from build123d import *

# Parameters (mm, degrees)
F1_DEPTH = 30
F3_R     = 3


# Not quite as in the source:
# - a feature of the source that left no trace in its solid (it failed there, or was rolled back) is left out


with BuildPart() as f1:
    # F0 (on Top) → F1 (new body)
    with BuildSketch(Plane.XY):
        with BuildLine():
            ThreePointArc((-37.25, 36.5), (-27.8459144936, 7.7690354349), (0, -4))
            ThreePointArc((0, -4), (26.5127811208, 8.5143386541), (35.25, 36.5))
            Line((35.25, 36.5), (-37.25, 36.5))
        make_face()
        with BuildLine():
            ThreePointArc((0, 0), (-23.5433609961, 9.1719845194), (-33.25, 32.5))
            Line((-33.25, 32.5), (31.25, 32.5))
            ThreePointArc((31.25, 32.5), (22.2476477305, 9.8820694899), (0, 0))
        make_face(mode=Mode.SUBTRACT)
    extrude(amount=F1_DEPTH)

    # F3
    f3_edges = [f1.edges().sort_by_distance(p)[0] for p in [
        (-1, 36.5, 0),
        (-1, -4.013711, 0),
        (-37.25, 36.5, 15),
        (35.25, 36.5, 15),
        (-1, 36.5, 30),
        (-1, -4.013711, 30),
    ]]
    fillet(f3_edges, radius=F3_R)


solid = f1.part
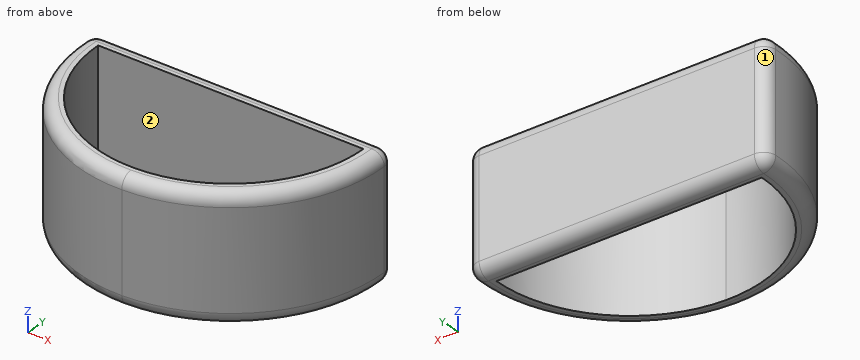
Verification items for the finished model (mm, model axes). Face numbers are marked on the shaded views. Give positions to 0.01 mm unless a question says otherwise; leave off trailing zeros. Loops run counter-clockwise (first coordinate to the right, second up) from the corner with the lowest first, then second, coordinate; pieces in that order, holes last.
1. Go/stop test with flat-tipped pins: P1, Ø4, axis at x = -18.5, z = 7, coming from the -Y side; P2, Ø2, axis at x = 26.5, y = 18, coming from the +Z side (1 decimal); P3, Ø2, axis at x = 15, y = 1.5, coming from the +Z side; P4, Ø3, axis at y = 29.5, z = 6, coming from the +X side. Record where each tip stops, or that it passes through.
Derived:
P1: stops at y = -0.56
P2: passes through
P3: stops at z = 29.98
P4: stops at x = 35.45
2. Release check for a two-part mould opening along Y. For the marked faces 1 and 2 record: +Y half, -Y half, draft (parallel to the pull), parting line (faces both ways), or undercut.
Derived:
face 1: +Y half
face 2: undercut
3. Material ranges on probe 1 along X at (y, z) = (9, 6); probe 2 along X at (y, z) = (3.5, 12.25); probe 3 along Y at (x, z) = (27.5, 16), recorded low to high.
Derived:
probe 1: x = -28.93 to -23.37, 21.37 to 26.93
probe 2: x = -23.17 to -15.64, 13.64 to 21.17
probe 3: y = 9.7 to 17.14, 32.5 to 36.5
4. Cross-section at A-A on z = 10.75. Record the cut outline in (x, y), and give its area (3 significant figures).
Derived:
outline: (-37.46, 33.59) arc R36.47 ccw (long way) to (35.46, 33.59) arc R3 ccw to (32.46, 36.5) - (-34.46, 36.5) arc R3 ccw to start; hole (-33.25, 32.5) arc R32.25 ccw (long way) to (31.25, 32.5) - close
area: 730 mm2
